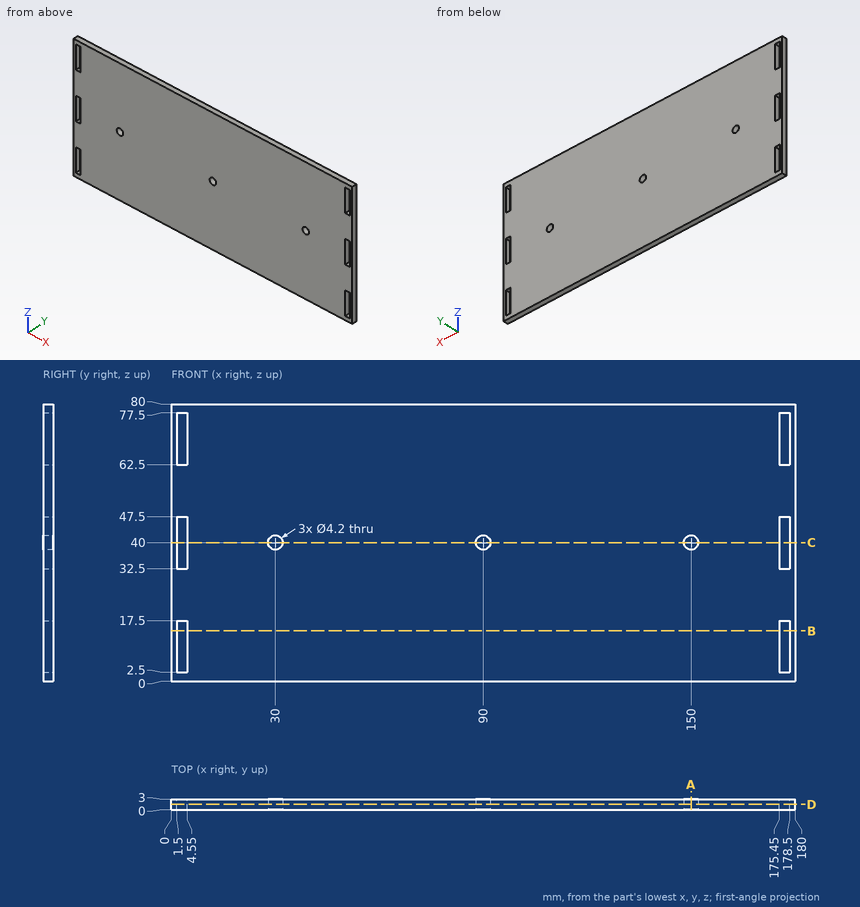
Design review of the part shown in the three views and the two pictorial views. Dimensions are in mm from the part's minimum x, y and z. Round coordinates to 2 decimals unless told otherwise and drop trailing zeros. Write each loop counter-clockwise with the first axis right and the second up, starting at its lowest first coordinate (ties: lowest second). Pieces come first, ordered by that corner, then holes. Notation, with made-up numbers: (18, 53.25) - (54, 53.25) arc R27 cw to (54, 85.25) - close; hole circle Ø9 at (13, -22.75). An arc over 180 degrees is marked (long way). Write item = value, one per line. Start each with the question number.
1. Consider section D-D on y = 1.5. Give the number of separate pieces and of enclosed holes in the cut face, plus the area to 3 significant figures.
2. Wall thickness on L1, parallel to X at y = 2.4, z = 47; L2, parallel to X at y = 0.8, z = 40; L3, parallel to Z at x = 30, y = 1.6: over which ranges is each line inside the solid? List them lowest first.
3. Consider section B-B on z = 14.5. State the section outline as (x, y) points, plus the area to 3 significant figures.
4. Consider section C-C on z = 40. State the section outline as (x, y) points.
5. For pin 1 Ø1.5 at (y, z) = (1, 72) entering from -X, flat-tipped, find the tip position at first contact; note if it passes through.
6. Consider section A-A on x = 150. State the section outline as (y, z) points, plus the area to 3 significant figures.
Evaluation:
q1.separate_pieces = 1
q1.enclosed_holes = 9
q1.area = 14,100 mm2
q2.L1 = 0 to 1.5, 4.55 to 175.45, 178.5 to 180
q2.L2 = 0 to 1.5, 4.55 to 27.9, 32.1 to 87.9, 92.1 to 147.9, 152.1 to 175.45, 178.5 to 180
q2.L3 = 0 to 37.9, 42.1 to 80
q3.outline = (0, 0) - (1.5, 0) - (1.5, 3) - (0, 3) - close; (4.55, 0) - (175.45, 0) - (175.45, 3) - (4.55, 3) - close; (178.5, 0) - (180, 0) - (180, 3) - (178.5, 3) - close
q3.area = 522 mm2
q4.outline = (0, 0) - (1.5, 0) - (1.5, 3) - (0, 3) - close; (4.55, 0) - (27.9, 0) - (27.9, 3) - (4.55, 3) - close; (32.1, 0) - (87.9, 0) - (87.9, 3) - (32.1, 3) - close; (92.1, 0) - (147.9, 0) - (147.9, 3) - (92.1, 3) - close; (152.1, 0) - (175.45, 0) - (175.45, 3) - (152.1, 3) - close; (178.5, 0) - (180, 0) - (180, 3) - (178.5, 3) - close
q5.pin_1 = 0
q6.outline = (0, 0) - (3, 0) - (3, 37.9) - (0, 37.9) - close; (0, 42.1) - (3, 42.1) - (3, 80) - (0, 80) - close
q6.area = 227 mm2
